Geometry check sheet. Reference: the model listing, model coordinates, mm. A direction names the side the tool comes from. Round coordinates to 2 decimals unless told otherwise and drop trailing zeros. Loops run counter-clockwise (first coordinate to the right, second up) from the corner with the lowest first, then second, coordinate; pieces in that order, holes last. Notation, with made-up numbers: (-6, -19) - (18, -19) arc R33 cw to (18, 18) - close; hole circle Ø9 at (11.25, -27.5). An arc over 180 degrees is marked (long way). Answer in a Markdown table with one row per item. Add a question column.
```python
from build123d import *

# Parameters (mm, degrees)
F0_R     = 11
F0_R_2   = 9
F1_DEPTH = 8.5
F0_R_3   = 26.1
F2_DEPTH = 3.5
F0_R_4   = 30.1
F3_DEPTH = 8.5


with BuildPart() as f1:
    # F0 (on Front) → F1 (new body, symmetric)
    with BuildSketch(Plane.XZ):
        Circle(F0_R)
        Circle(F0_R_2, mode=Mode.SUBTRACT)
    extrude(amount=F1_DEPTH, both=True)

    # F0 (on Front) → F2 (join, symmetric)
    with BuildSketch(Plane.XZ):
        Circle(F0_R_3)
        Circle(F0_R, mode=Mode.SUBTRACT)
    extrude(amount=F2_DEPTH, both=True)

    # F0 (on Front) → F3 (join, symmetric)
    with BuildSketch(Plane.XZ):
        Circle(F0_R_4)
        Circle(F0_R_3, mode=Mode.SUBTRACT)
    extrude(amount=F3_DEPTH, both=True)


solid = f1.part
```
Q1. Cross-section at D-D, the plane x = -24. Enter the section's corners in (y, z), plus the area to 3 significant figures.
Q2. Cross-section at C-C, the plane y = -4.25. Enter the section's corners in (x, z).
Q3. Scan lines: line 1 (Z direction, x = 0, y = 6.9); line 2 (X direction, y = -5, z = -22); line 3 (Z direction, x = -18.5, y = 5.25). Record each from-to range of solid material in increasing order. Write a range as from..to.
Q4. Depth check by flat-ended pin: P1, Ø4, axis at x = -22.5, z = 2, coming from the +Y side; P2, Ø8, axis at y = -2.5, z = -8, coming from the +X side; P3, Ø4, axis at x = -23, y = -4, coming from the -Z side. Enter the tip coordinate at first touch or a pass-through.
Q5. Cross-section at A-A, the plane x = 0. Enter the section's corners in (y, z), plus the area to 3 significant figures.
Q6. Set-up check for faces 1 (the flat face through (-9, 8.5, 25)), 2 (the cylindrical face through (-2.38, 5.96, -10.74)), 3 (the cylindrical face through (-19.237, -5.965, 17.64)): record each of +Z, -Z, +X, -X, +Y, -Y from which the full face is reachable in a straight line by a thin tool's end or side.
Q7. Release check for a two-part mould opening along X. For faces 4 (the cylindrical face through (-6.525, -0.119, -29.384)), 5 (the flat face through (2, -8.5, -9)), 6 (the cylindrical face through (-19.237, 6.035, 17.64)) record: +X half, -X half, draft (parallel to the pull), parting line (faces both ways), or undercut.
Q8. Cross-section at B-B, the plane z = 0. Enter the section's corners in (x, y).
Check sheet entries:
| question | item | result |
|---|---|---|
| 1 | outline | (-8.5, -18.17) - (8.5, -18.17) - (8.5, -10.26) - (3.5, -10.26) - (3.5, 10.26) - (8.5, 10.26) - (8.5, 18.17) - (-8.5, 18.17) - (-8.5, 10.26) - (-3.5, 10.26) - (-3.5, -10.26) - (-8.5, -10.26) - close |
| 1 | area | 413 mm² |
| 2 | outline | circle Ø60.2 at (0, 0); circle Ø22 at (0, 0); hole circle Ø52.2 at (0, 0); hole circle Ø18 at (0, 0) |
| 3 | line 1 | -30.1..-26.1, -11..-9, 9..11, 26.1..30.1 |
| 3 | line 2 | -20.54..-14.04, 14.04..20.54 |
| 3 | line 3 | -23.74..-18.41, 18.41..23.74 |
| 4 | P1 | y = 3.5 |
| 4 | P2 | x = 29.83 |
| 4 | P3 | z = -21.56 |
| 5 | outline | (-8.5, -30.1) - (8.5, -30.1) - (8.5, -26.1) - (3.5, -26.1) - (3.5, -11) - (8.5, -11) - (8.5, -9) - (-8.5, -9) - (-8.5, -11) - (-3.5, -11) - (-3.5, -26.1) - (-8.5, -26.1) - close; (-8.5, 9) - (8.5, 9) - (8.5, 11) - (3.5, 11) - (3.5, 26.1) - (8.5, 26.1) - (8.5, 30.1) - (-8.5, 30.1) - (-8.5, 26.1) - (-3.5, 26.1) - (-3.5, 11) - (-8.5, 11) - close |
| 5 | area | 415 mm² |
| 6 | face 1 | +Z, -Z, +X, -X, +Y |
| 6 | face 2 | +Y |
| 6 | face 3 | -Y |
| 7 | face 4 | parting line |
| 7 | face 5 | draft |
| 7 | face 6 | undercut |
| 8 | outline | (-30.1, -8.5) - (-26.1, -8.5) - (-26.1, -3.5) - (-11, -3.5) - (-11, -8.5) - (-9, -8.5) - (-9, 8.5) - (-11, 8.5) - (-11, 3.5) - (-26.1, 3.5) - (-26.1, 8.5) - (-30.1, 8.5) - close; (9, -8.5) - (11, -8.5) - (11, -3.5) - (26.1, -3.5) - (26.1, -8.5) - (30.1, -8.5) - (30.1, 8.5) - (26.1, 8.5) - (26.1, 3.5) - (11, 3.5) - (11, 8.5) - (9, 8.5) - close |
